```python
from build123d import *

# Parameters (mm, degrees)
BOSS_EXTRUDE1_DEPTH = 6.35
CUT_EXTRUDE1_DEPTH  = 7.35


with BuildPart() as part:
    # Sketch1 → Boss-Extrude1 (new body)
    with BuildSketch(Plane(origin=(0, 0, 0), x_dir=(1, 0, 0), z_dir=(0, 1, 0))):
        Polygon((67.038031479, -56.883887939), (50.857913673, 145.670904124), (-146.783072598, 192.87557069), (-252.751801878, 19.494866992), (-120.603092047, -134.864967453), align=None)
    extrude(amount=BOSS_EXTRUDE1_DEPTH)

    # Sketch2 → Cut-Extrude1 (cut, through all)
    with BuildSketch(Plane(origin=(0, 6.35, 0), x_dir=(1, 0, 0), z_dir=(0, 1, 0))):
        Polygon((-87.85729012, -114.379729934), (-64.40214968, -104.632094995), (-61.965240945, -110.495880105), (-85.420381385, -120.243515044), align=None)
        Polygon((-38.510100504, -100.748245166), (-15.054960063, -91.000610226), (-17.491868798, -85.136825116), (-40.947009239, -94.884460055), align=None)
        Polygon((8.400180377, -81.252975287), (31.855320818, -71.505340348), (29.418412083, -65.641555238), (5.963271643, -75.389190177), align=None)
        Polygon((-223.150173958, -5.317954784), (-206.631585229, -24.61293409), (-211.455330056, -28.742581272), (-227.973918785, -9.447601966), align=None)
        Polygon((-194.936741327, -48.037560577), (-190.112996501, -43.907913395), (-173.594407772, -63.202892701), (-178.418152598, -67.332539883), align=None)
        Polygon((-161.899563869, -86.627519189), (-157.075819043, -82.497872006), (-140.557230314, -101.792851312), (-145.38097514, -105.922498494), align=None)
        Polygon((-161.234062348, 157.055165957), (-174.480153508, 135.382577994), (-179.898300498, 138.694100784), (-166.652209338, 160.366688747), align=None)
        Polygon((-193.144391658, 117.021512822), (-187.726244668, 113.709990032), (-200.972335828, 92.03740207), (-206.390482818, 95.34892486), align=None)
        Polygon((-219.636573978, 73.676336898), (-214.218426988, 70.364814108), (-227.464518148, 48.692226145), (-232.882665138, 52.003748935), align=None)
        Polygon((12.325082917, 148.345498284), (-12.380040367, 154.246081605), (-10.904894536, 160.422362426), (13.800228747, 154.521779105), align=None)
        Polygon((-35.61001782, 166.322945747), (-37.085163651, 160.146664926), (-61.790286935, 166.047248246), (-60.315141104, 172.223529067), align=None)
        Polygon((-85.020264388, 178.124112388), (-86.495410219, 171.947831567), (-111.200533502, 177.848414888), (-109.725387672, 184.024695709), align=None)
        Polygon((57.674422139, -19.410493109), (55.651907413, 5.908855899), (61.981744665, 6.41448458), (64.004259391, -18.904864428), align=None)
        Polygon((59.959229939, 31.733833588), (53.629392687, 31.228204907), (51.606877961, 56.547553915), (57.936715213, 57.053182596), align=None)
        Polygon((55.914200488, 82.372531604), (49.584363236, 81.866902923), (47.56184851, 107.186251931), (53.891685762, 107.691880612), align=None)
    extrude(amount=-CUT_EXTRUDE1_DEPTH, mode=Mode.SUBTRACT)


solid = part.part
```
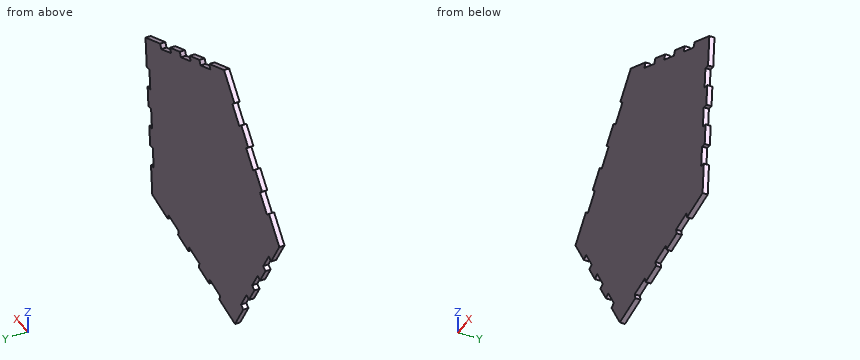
Source: CAD feature listing. Evaluate the final solid. Frame: model axes, mm. Round coordinates to 2 decimals unless told otherwise and drop trailing zeros. Loops run counter-clockwise (first coordinate to the right, second up) from the corner with the lowest first, then second, coordinate; pieces in that order, holes last.
1. Contact query for flat-ended pins moving along their axis: pin 1 (2 mm diameter, centred on x = -76.5, y = 5, fed in from +Z); pin 2 (1.5 mm diameter, centred on y = 5, z = 21.5, fed in from -X); pin 3 (1.5 mm diameter, centred on x = -55, y = 3.5, fed in from -Z). Output: stop coordinate, or through.
2. Ray query, L1, parallel to X at y = 0.5, z = -135.5; L2, parallel to Z at x = -209.5, y = 3; L3, parallel to Z at x = -39, y = 2. Return the intervals inside material, ascending.
3. Section query B-B on z = 0. Output: boundary loops of the cut face in (x, y), and give its area (3 significant figures).
4. Section query A-A on x = -126. Output: boundary loops of the cut face in (y, z).
Answers below:
1. pin 1: stops at z = 110.08
1. pin 2: stops at x = -209.94
1. pin 3: stops at z = -164.6
2. L1: x = -181.85 to -174.67, -174.41 to 51.67
2. L2: z = -90.26 to 21.26, 27.07 to 31.03
2. L3: z = -160.6 to 94.08, 99.57 to 100.95
3. outline: (-236.06, 0) - (56.12, 0) - (56.12, 6.35) - (-236.06, 6.35) - close
3. area: 1,860 mm2
4. outline: (0, -187.91) - (6.35, -187.91) - (6.35, 128.56) - (0, 128.56) - close
